The model under review builds one solid part; all positions refer to its coordinate system, in mm. Face numbers are marked on the shaded views. Coordinates: 2 decimals unless noted, no trailing zeros. Loops run counter-clockwise (first coordinate to the right, second up) from the corner with the lowest first, then second, coordinate; pieces in that order, holes last. Notation, with made-up numbers: M 7,79 L 22,79 A35 cw 22,111 Z; hole C 71.25,-5.75 d7. An arc over 180 degrees is marked long. Write item = value, one per line. Start each with the question number.
Q1. Clearance check with flat-ended pins moving along their axes: pin 1 Ø5 at (y, z) = (-40.5, 10.5) entering from -X; pin 2 Ø3.5 at (x, y) = (14.85, 7) entering from +Z; pin 3 Ø1 at (x, z) = (3.5, 1) entering from +Y. State where each tip first meets the part, or that it passes through.
Q2. We need section A-A on y = 12.5. Give the boundary of the cut face in (x, z) (3 decimals), and give its area (3 significant figures).
Q3. Mouldability with a two-part tool opening along Z and no side actions: class the marked faces 1, 2, 3 and 4 as released by +Z, released by -Z, zero draft, split by the parting line, or undercut.
Q4. Wall thickness on probe 1 along Y at (x, z) = (5.25, 1.5); probe 2 along Y at (x, z) = (-7.5, 13); probe 3 along Z at (x, y) = (3, -23): over which ranges is each line inside the solid? List them lowest first.
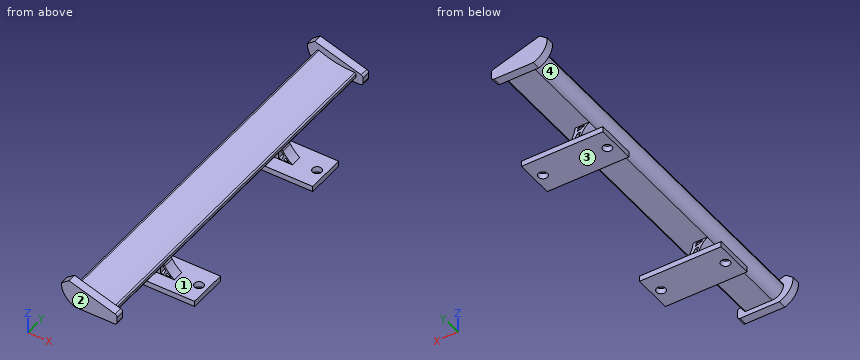
from build123d import *

# Parameters (mm, degrees)
CROQUIS1_W                = 29.1
CROQUIS1_H                = 14
CROQUIS1_R                = 1.625
SALIENTE_EXTRUIR1_DEPTH   = 2
SALIENTE_EXTRUIR1_2_DEPTH = 2
CROQUIS2_W                = 8
CROQUIS2_H                = 8
SALIENTE_EXTRUIR2_DEPTH   = 7
CROQUIS3_W                = 28
CROQUIS3_H                = 135.79635
SALIENTE_EXTRUIR3_DEPTH   = 8
CORTAR_EXTRUIR1_START     = -135.79635
CORTAR_EXTRUIR1_DEPTH     = 135.79635
REDONDEO1_R               = 0.5
REDONDEO2_R               = 0.5
CROQUIS5_W                = 2
CROQUIS5_H                = 32
CROQUIS5_H_2              = 55.79635
CORTAR_EXTRUIR2_DEPTH     = 8
SALIENTE_EXTRUIR4_DEPTH   = 3
REDONDEO4_R               = 1
SALIENTE_EXTRUIR5_DEPTH   = 3
CORTAR_EXTRUIR4_START     = -71.79635
CORTAR_EXTRUIR4_DEPTH     = 71.79635
SALIENTE_EXTRUIR7_START   = -8
SALIENTE_EXTRUIR7_DEPTH   = 8
SALIENTE_EXTRUIR8_START   = -8
SALIENTE_EXTRUIR8_DEPTH   = 8
CORTAR_EXTRUIR5_START     = -71.79635
CORTAR_EXTRUIR5_DEPTH     = 71.79635
REDONDEO5_R               = 4
CORTAR_EXTRUIR6_START     = -21.901142
CROQUIS15_W               = 9
CROQUIS15_H               = 2
CORTAR_EXTRUIR6_DEPTH     = 14.356142
CORTAR_EXTRUIR7_START     = -103.79635
CROQUIS16_W               = 5.770605939
CROQUIS16_H               = 2
CROQUIS16_W_2             = 12.752116736
CORTAR_EXTRUIR7_DEPTH     = 129.79635
CROQUIS17_W               = 9.132432918
CROQUIS17_H               = 14
CROQUIS17_R               = 1.625
CROQUIS17_W_2             = 9.390289757
SALIENTE_EXTRUIR9_DEPTH   = 2


with BuildPart() as part:
    # Croquis1 → Saliente-Extruir1 (new body)
    with BuildSketch(Plane.XY):
        with Locations((0, -56.79635)):
            Rectangle(CROQUIS1_W, CROQUIS1_H)
        with Locations((11.49, -56.79635)):
            Circle(CROQUIS1_R, mode=Mode.SUBTRACT)
        with Locations((-11.5, -56.79635)):
            Circle(CROQUIS1_R, mode=Mode.SUBTRACT)
    extrude(amount=SALIENTE_EXTRUIR1_DEPTH)



with BuildPart() as body_2:
    # Croquis1 → Saliente-Extruir1 2 (new body)
    with BuildSketch(Plane.XY):
        with Locations((0, 7)):
            Rectangle(CROQUIS1_W, CROQUIS1_H)
        with Locations((-11.5, 7)):
            Circle(CROQUIS1_R, mode=Mode.SUBTRACT)
        with Locations((11.49, 7)):
            Circle(CROQUIS1_R, mode=Mode.SUBTRACT)
    extrude(amount=SALIENTE_EXTRUIR1_2_DEPTH)


with BuildPart() as part_1:
    add(part.part)

    add(body_2.part)  # Saliente-Extruir2 merges body 2
    # Croquis2 → Saliente-Extruir2 (add)
    with BuildSketch(Plane.XY.offset(2)):
        with Locations((-0.005, 7)):
            Rectangle(CROQUIS2_W, CROQUIS2_H)
        with Locations((-0.005, -56.79635)):
            Rectangle(CROQUIS2_W, CROQUIS2_H)
    extrude(amount=SALIENTE_EXTRUIR2_DEPTH)

    # Croquis3 → Saliente-Extruir3 (add)
    with BuildSketch(Plane.XY.offset(9)):
        with Locations((-0.005, -24.898175)):
            Rectangle(CROQUIS3_W, CROQUIS3_H)
    extrude(amount=SALIENTE_EXTRUIR3_DEPTH)

    # Croquis4 → Cortar-Extruir1 (cut)
    with BuildSketch(Plane(origin=(0, 43, 0), x_dir=(1, 0, 0), z_dir=(0, 1, 0)).offset(CORTAR_EXTRUIR1_START)):
        with BuildLine():
            Line((3.995, -9), (3.995, -11))
            Line((3.995, -11), (6.995, -11))
            Line((6.995, -11), (6.995, -13))
            ThreePointArc((6.995, -13), (-0.186595872, -13.652552595), (-7.005, -16))
            Line((-7.005, -16), (-7.005, -13))
            Line((-7.005, -13), (-7.005, -11))
            Line((-7.005, -11), (-4.005, -11))
            Line((-4.005, -11), (-4.005, -9))
            Line((-4.005, -9), (-14.005, -9))
            Line((-14.005, -9), (-14.005, -17))
            Line((-14.005, -17), (13.995, -17))
            Line((13.995, -17), (13.995, -9))
            Line((13.995, -9), (3.995, -9))
        make_face()
    extrude(amount=CORTAR_EXTRUIR1_DEPTH, mode=Mode.SUBTRACT)

    # Redondeo1
    redondeo1_edges = [part_1.edges().sort_by_distance(p)[0] for p in [
        (6.995, -24.898175, 13),
        (6.995, -24.898175, 11),
    ]]
    fillet(redondeo1_edges, radius=REDONDEO1_R)

    # Redondeo2
    redondeo2_edges = [part_1.edges().sort_by_distance(p)[0] for p in [
        (-7.005, -24.898175, 16),
    ]]
    fillet(redondeo2_edges, radius=REDONDEO2_R)

    # Croquis5 → Cortar-Extruir2 (cut)
    with BuildSketch(Plane.ZY.offset(4.005)):
        with Locations((10, 27)):
            Rectangle(CROQUIS5_W, CROQUIS5_H)
        with Locations((10, -24.898175)):
            Rectangle(CROQUIS5_W, CROQUIS5_H_2)
        with Locations((10, -76.79635)):
            Rectangle(CROQUIS5_W, CROQUIS5_H)
    extrude(amount=-CORTAR_EXTRUIR2_DEPTH, mode=Mode.SUBTRACT)

    # Croquis6 → Saliente-Extruir4 (add)
    with BuildSketch(Plane(origin=(0, 43, 0), x_dir=(1, 0, 0), z_dir=(0, 1, 0))):
        with BuildLine():
            Line((9.457278185, -12.908301876), (-7.759178779, -18.474170155))
            Line((-7.759178779, -18.474170155), (-10.447776168, -16.398761645))
            ThreePointArc((-10.447776168, -16.398761645), (-9.123523754, -12.023120399), (-5.505, -9.229168607))
            Line((-5.505, -9.229168607), (9.457278185, -9.229168607))
            Line((9.457278185, -9.229168607), (9.457278185, -12.908301876))
        make_face()
    extrude(amount=-SALIENTE_EXTRUIR4_DEPTH)

    # Redondeo4
    redondeo4_edges = [part_1.edges().sort_by_distance(p)[0] for p in [
        (9.457278185, 41.5, 9.229168607),
        (9.457278185, 41.5, 12.908301876),
    ]]
    fillet(redondeo4_edges, radius=REDONDEO4_R)

    # Croquis7 → Saliente-Extruir5 (add)
    with BuildSketch(Plane.XZ.offset(92.79635)):
        with BuildLine():
            Line((-7.759178779, 18.474170155), (8.76489024, 13.132142363))
            ThreePointArc((8.76489024, 13.132142363), (9.265860913, 12.769013006), (9.457278185, 12.180630501))
            Line((9.457278185, 12.180630501), (9.457278185, 10.229168607))
            ThreePointArc((9.457278185, 10.229168607), (9.164384967, 9.522061826), (8.457278185, 9.229168607))
            Line((8.457278185, 9.229168607), (-5.505, 9.229168607))
            ThreePointArc((-5.505, 9.229168607), (-9.123523754, 12.023120399), (-10.447776168, 16.398761645))
            Line((-10.447776168, 16.398761645), (-7.759178779, 18.474170155))
        make_face()
    extrude(amount=-SALIENTE_EXTRUIR5_DEPTH)

    # Croquis11 → Cortar-Extruir4 (cut)
    with BuildSketch(Plane(origin=(0, 11, 0), x_dir=(1, 0, 0), z_dir=(0, 1, 0)).offset(CORTAR_EXTRUIR4_START)):
        with BuildLine():
            Line((-4.005, -11), (-3.005, -11))
            ThreePointArc((-3.005, -11), (-0.024192095, -6.993590584), (0, -2))
            Line((0, -2), (-4.005, -2))
            Line((-4.005, -2), (-4.005, -11))
        make_face()
        with BuildLine():
            Line((3.995, -11), (1.995, -11))
            ThreePointArc((1.995, -11), (2.742037907, -8.281661906), (3.995, -5.756287949))
            Line((3.995, -5.756287949), (3.995, -11))
        make_face()
    extrude(amount=CORTAR_EXTRUIR4_DEPTH, mode=Mode.SUBTRACT)

    # Croquis12 → Saliente-Extruir7 (add)
    with BuildSketch(Plane(origin=(0, 11, 0), x_dir=(1, 0, 0), z_dir=(0, 1, 0)).offset(SALIENTE_EXTRUIR7_START)):
        with BuildLine():
            Line((3.995, -2), (7.351142184, -2))
            ThreePointArc((7.351142184, -2), (5.510724817, -3.733091947), (3.995, -5.756287949))
            Line((3.995, -5.756287949), (3.995, -2))
        make_face()
    extrude(amount=SALIENTE_EXTRUIR7_DEPTH)

    # Croquis13 → Saliente-Extruir8 (add)
    with BuildSketch(Plane.XZ.offset(60.79635).offset(SALIENTE_EXTRUIR8_START)):
        with BuildLine():
            Line((3.995, 5.756287949), (3.995, 2))
            Line((3.995, 2), (7.351142184, 2))
            ThreePointArc((7.351142184, 2), (5.510724817, 3.733091947), (3.995, 5.756287949))
        make_face()
    extrude(amount=SALIENTE_EXTRUIR8_DEPTH)

    # Croquis14 → Cortar-Extruir5 (cut)
    with BuildSketch(Plane(origin=(0, 11, 0), x_dir=(1, 0, 0), z_dir=(0, 1, 0)).offset(CORTAR_EXTRUIR5_START)):
        Polygon((6.21693803, -2.324666095), (4.927658189, -3.565597942), (4.331366262, -2.566406065), align=None)
        Polygon((3.493334365, -2.324666095), (2.47802649, -2.324666095), (2.47802649, -6.595405569), (4.331366262, -4.210237863), align=None)
        Polygon((1.235275319, -5.075942388), (2.002667058, -7.167084876), (1.235275319, -8.490835625), (0.160926885, -8.68268356), align=None)
        Polygon((0.97157316, -10.515246809), (-1.531379092, -10.515246809), (1.235275319, -9.257285848), align=None)
    extrude(amount=CORTAR_EXTRUIR5_DEPTH, mode=Mode.SUBTRACT)

    # Redondeo5
    redondeo5_edges = [part_1.edges().sort_by_distance(p)[0] for p in [
        (-7.005, -24.898175, 11),
    ]]
    fillet(redondeo5_edges, radius=REDONDEO5_R - 0.0001)  # a hair under: the kernel refuses the full size

    # Croquis15 → Cortar-Extruir6 (cut)
    with BuildSketch(Plane.ZY.offset(14.55).offset(CORTAR_EXTRUIR6_START)):
        with Locations((6.5, 10)):
            Rectangle(CROQUIS15_W, CROQUIS15_H)
        with Locations((6.5, 4)):
            Rectangle(CROQUIS15_W, CROQUIS15_H)
        with Locations((6.5, -53.79635)):
            Rectangle(CROQUIS15_W, CROQUIS15_H)
        with Locations((6.5, -59.79635)):
            Rectangle(CROQUIS15_W, CROQUIS15_H)
    extrude(amount=CORTAR_EXTRUIR6_DEPTH, mode=Mode.SUBTRACT)

    # Croquis16 → Cortar-Extruir7 (cut)
    with BuildSketch(Plane(origin=(0, 14, 0), x_dir=(1, 0, 0), z_dir=(0, 1, 0)).offset(CORTAR_EXTRUIR7_START)):
        with Locations((11.664697031, -1)):
            Rectangle(CROQUIS16_W, CROQUIS16_H)
        with Locations((-8.173941632, -1)):
            Rectangle(CROQUIS16_W_2, CROQUIS16_H)
    extrude(amount=CORTAR_EXTRUIR7_DEPTH, mode=Mode.SUBTRACT)

    # Croquis17 → Saliente-Extruir9 (add)
    # profile 1 of 4: a face of its own
    with BuildSketch(Plane.XY.offset(2)):
        with Locations((13.34561052, 7)):
            Rectangle(CROQUIS17_W, CROQUIS17_H)
        with Locations((14.851826979, 7)):
            Circle(CROQUIS17_R, mode=Mode.SUBTRACT)
    # profile 2 of 4: a face of its own
    with BuildSketch(Plane.XY.offset(2)):
        with Locations((-6.493028143, 7)):
            Rectangle(CROQUIS17_W_2, CROQUIS17_H)
        with Locations((-8.138173021, 7)):
            Circle(CROQUIS17_R, mode=Mode.SUBTRACT)
    # profile 3 of 4: a face of its own
    with BuildSketch(Plane.XY.offset(2)):
        with Locations((-6.493028143, -56.79635)):
            Rectangle(CROQUIS17_W_2, CROQUIS17_H)
        with Locations((-8.138173021, -56.79635)):
            Circle(CROQUIS17_R, mode=Mode.SUBTRACT)
    # profile 4 of 4: a face of its own
    with BuildSketch(Plane.XY.offset(2)):
        with Locations((13.34561052, -56.79635)):
            Rectangle(CROQUIS17_W, CROQUIS17_H)
        with Locations((14.851826979, -56.79635)):
            Circle(CROQUIS17_R, mode=Mode.SUBTRACT)
    extrude(amount=-SALIENTE_EXTRUIR9_DEPTH)


solid = part_1.part
Returned:
q1.pin_1 = -6.47
q1.pin_2 = 2
q1.pin_3 = 14
q2.outline = M -11.188,0 L 17.912,0 L 17.912,2 L -11.188,2 Z; M -7.005,15 A4 ccw -3.005,11 L 6.495,11 A0.5 ccw 6.995,11.5 L 6.995,12.489 A0.5 ccw 6.489,12.989 A30 cw -6.298,15.668 A0.5 ccw -7.005,15.213 Z
q2.area = 95.2 mm^2
q3.face_1 = undercut
q3.face_2 = zero draft
q3.face_3 = released by -Z
q3.face_4 = undercut
q4.probe_1 = -63.8 to -49.8, 0 to 14
q4.probe_2 = -92.8 to -89.8, 40 to 43
q4.probe_3 = 11 to 13.15
